from build123d import *

# Parameters (mm, degrees)
SKETCH1_R           = 42.725
SKETCH1_R_2         = 37.875
BOSS_EXTRUDE1_DEPTH = 196.5
SKETCH2_R           = 9.94
CUT_EXTRUDE1_DEPTH  = 206.57991451
SKETCH4_R           = 7.5
CUT_EXTRUDE2_DEPTH  = 206.579914647


with BuildPart() as part:
    # Sketch1 → Boss-Extrude1 (new body)
    with BuildSketch(Plane(origin=(0, 0, 0), x_dir=(1, 0, 0), z_dir=(0, 1, 0))):
        with Locations(Location((0, 0, 0), (0, 0, 270))):
            Circle(SKETCH1_R)
        with Locations(Location((0, 0, 0), (0, 0, 270))):
            Circle(SKETCH1_R_2, mode=Mode.SUBTRACT)
    extrude(amount=BOSS_EXTRUDE1_DEPTH)

    # Sketch2 → Cut-Extrude1 (cut, through all)
    with BuildSketch(Plane(origin=(0, 0, 0), x_dir=(0, 0, -1), z_dir=(1, 0, 0))):
        with Locations(Location((0, 131.8, 0), (0, 0, 180))):
            Circle(SKETCH2_R)
        with Locations(Location((0, 80.8, 0), (0, 0, 180))):
            Circle(SKETCH2_R)
        with Locations(Location((0, 29.8, 0), (0, 0, 180))):
            Circle(SKETCH2_R)
    extrude(amount=CUT_EXTRUDE1_DEPTH, mode=Mode.SUBTRACT)

    # Sketch4 → Cut-Extrude2 (cut, through all)
    with BuildSketch(Plane(origin=(0, 0, 0), x_dir=(0, 0, -1), z_dir=(1, 0, 0))):
        with Locations((0, 106.3)):
            Circle(SKETCH4_R)
    extrude(amount=-CUT_EXTRUDE2_DEPTH, mode=Mode.SUBTRACT)


solid = part.part
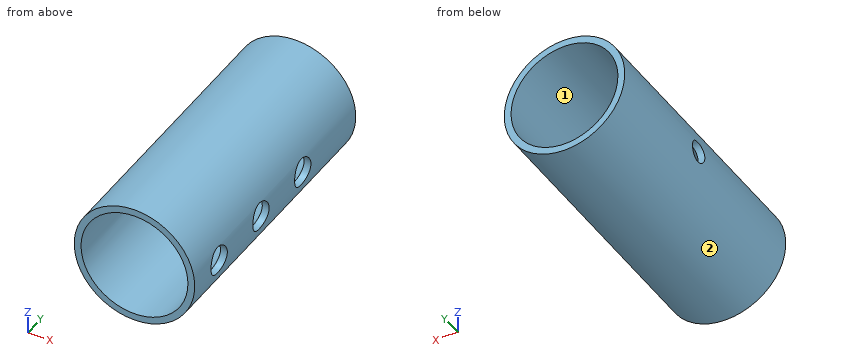
For this review, take the finished solid that the model builds, in its own axes (mm). Face numbers are marked on the shaded views. Round coordinates to 2 decimals unless told otherwise and drop trailing zeros. Order: outer loops, then holes, each group sorted by start corner. A loop starts at its lowest first (then second) coordinate and runs counter-clockwise, first axis right, second up. Notation, with made-up numbers: (48, 2) -> (68, 2) arc R23 ccw to (68, 26) -> close; hole circle Ø3 at (73.5, 58). An arc over 180 degrees is marked (long way). Put each result on its own line as item: value.
Q1. Add section C-C on z = -16. Write out the cut boundary in (x, y).
Check result:
outline: (-39.62, 0) -> (-34.33, 0) -> (-34.33, 196.5) -> (-39.62, 196.5) -> close; (34.33, 0) -> (39.62, 0) -> (39.62, 196.5) -> (34.33, 196.5) -> close
Q2. Insertion check: pin 1 Ø18 at (y, z) = (80.8, 0) entering from +X; pin 2 Ø1 at (x, z) = (34, -10.5) entering from -Y; pin 3 Ø4 at (x, y) = (12.5, 154.5) entering from -Z; pin 4 Ø1 at (x, y) = (-24.5, 133.5) entering from +Z. Each pin has a flat end and moves straight along its axis. Give the tip position at first contact, or say it passes through.
Check result:
pin 1: x = -36.79
pin 2: through
pin 3: z = -41.41
pin 4: z = 35.35
Q3. Mouldability with a two-part tool opening along Z and no side actions: class the marked faces 1 and 2 as pulls with the +Z half, pulls with the -Z half, needs draft (parallel to the pull), parting line crosses it, or undercut.
Check result:
face 1: undercut
face 2: parting line crosses it
Q4. Add section A-A on x = 0. Write out the cut boundary in (y, z) (3 decimals).
Check result:
outline: (0, -42.725) -> (196.5, -42.725) -> (196.5, -37.875) -> (0, -37.875) -> close; (0, 37.875) -> (196.5, 37.875) -> (196.5, 42.725) -> (0, 42.725) -> close
Q5. Add section D-D on y = 148. Write out the cut boundary in (x, z) (3 decimals).
Check result:
outline: circle Ø85.45 at (0, 0); hole circle Ø75.75 at (0, 0)
Q6. For probe 1 along Y at (x, z) = (41, 0); probe 2 along X at (y, z) = (65, 0) (3 decimals); probe 3 along X at (y, z) = (130, -0.5), list the stretches that pass through material, from the lowest coordinate up. Write a range as [from, to].
Check result:
probe 1: [0, 19.86], [39.74, 70.86], [90.74, 121.86], [141.74, 196.5]
probe 2: [-42.725, -37.875], [37.875, 42.725]
probe 3: [-42.72, -37.87]
Q7. Add section B-B on z = 0. Write out the cut boundary in (x, y) (3 decimals), plus the area to 3 significant figures.
Check result:
outline: (-42.725, 0) -> (-37.875, 0) -> (-37.875, 98.8) -> (-42.725, 98.8) -> close; (-42.725, 113.8) -> (-37.875, 113.8) -> (-37.875, 196.5) -> (-42.725, 196.5) -> close; (37.875, 0) -> (42.725, 0) -> (42.725, 19.86) -> (37.875, 19.86) -> close; (37.875, 39.74) -> (42.725, 39.74) -> (42.725, 70.86) -> (37.875, 70.86) -> close; (37.875, 90.74) -> (42.725, 90.74) -> (42.725, 121.86) -> (37.875, 121.86) -> close; (37.875, 141.74) -> (42.725, 141.74) -> (42.725, 196.5) -> (37.875, 196.5) -> close
area: 1,540 mm2
